Work out the finished part from the listing and answer in its coordinate system (mm). Round coordinates to 2 decimals unless told otherwise and drop trailing zeros. Loops run counter-clockwise (first coordinate to the right, second up) from the corner with the lowest first, then second, coordinate; pieces in that order, holes last. Notation, with made-up numbers: (-6.5, 71) - (43.5, 71) arc R15 cw to (43.5, 77) - close; hole circle Ø3 at (83, -25). An arc over 180 degrees is marked (long way). Use CSV: the item, a comma, the result in double quotes. Start each with the question number.
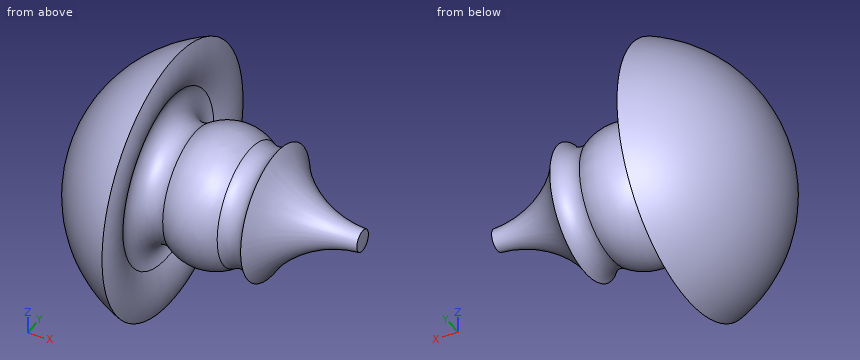
from build123d import *
from build123d.topology import SkipClean

# Parameters (mm, degrees)
SKETCH_3_R = 111.666392741


with BuildPart() as part:
    # 草圖1 → 旋轉1 (revolve)
    with BuildSketch(Plane.XY):
        with BuildLine():
            Line((0, 150), (0, -150))
            ThreePointArc((0, -150), (150, 0), (0, 150))
        make_face()
    revolve(axis=Axis((0, 150, 0), (0, -1, 0)))

    # 草圖2 → 除料-旋轉1 (revolve, cut)
    with SkipClean():  # the faces are left unmerged after this step: merging them gives an invalid solid
        with BuildSketch(Plane.XY, mode=Mode.PRIVATE) as cut_revolve_1_sk:
            with BuildLine():
                ThreePointArc((56.641005887, 148.905996075), (47.888974491, 120), (56.641005887, 91.094003925))
                ThreePointArc((56.641005887, 91.094003925), (54.142135624, 65.857864376), (28.905996075, 63.358994113))
                ThreePointArc((28.905996075, 63.358994113), (0, 72.111025509), (-28.905996075, 63.358994113))
                ThreePointArc((-28.905996075, 63.358994113), (-54.142135624, 65.857864376), (-56.641005887, 91.094003925))
                ThreePointArc((-56.641005887, 91.094003925), (-47.888974491, 120), (-56.641005887, 148.905996075))
                ThreePointArc((-56.641005887, 148.905996075), (-54.142135624, 174.142135624), (-28.905996075, 176.641005887))
                ThreePointArc((-28.905996075, 176.641005887), (0, 167.888974491), (28.905996075, 176.641005887))
                ThreePointArc((28.905996075, 176.641005887), (54.142135624, 174.142135624), (56.641005887, 148.905996075))
            make_face()
        revolve(cut_revolve_1_sk.sketch.rotate(Axis((0, 0, 0), (1, 0, 0)), 90), axis=Axis((0, 0, 0), (1, 0, 0)), mode=Mode.SUBTRACT)

    # 草圖3 → 除料-旋轉4 (revolve, cut)
    with SkipClean():  # the faces are left unmerged after this step: merging them gives an invalid solid
        with BuildSketch(Plane.XY, mode=Mode.PRIVATE) as cut_revolve_4_sk:
            with Locations((154.97116456, 123.10538907)):
                Circle(SKETCH_3_R)
        revolve(cut_revolve_4_sk.sketch.rotate(Axis((0, 0, 0), (1, 0, 0)), 90), axis=Axis((0, 0, 0), (1, 0, 0)), mode=Mode.SUBTRACT)


solid = part.part
Item 1: Find the intervals of material crossed by probe 1 along X at (y, z) = (4.5, 67.5); probe 2 along X at (y, z) = (1, 3); probe 3 along Y at (x, z) = (-16, 1), in increasing order. Write a range as [from, to].
Item 2: A cutting plane is placed at B-B (x = 48). Determine the outline of the cut face in (y, z).
Item 3: Each of these flat-tipped pins is pushed along its axis until it touches: pin 1 Ø4 at (x, z) = (-21.5, 29) entering from -Y; pin 2 Ø10 at (x, y) = (-13.5, -16.5) entering from -Z; pin 3 Ø8 at (x, z) = (-66.5, -39.5) entering from +Y. Where does it stop, or does it pass through?
Item 4: A cutting plane is placed at A-A (x = -40). Determine the outline of the cut face in (y, z), plus the area to 3 significant figures.
Result sheet:
1,probe 1,"[-133.88, -55.73], [-21.1, 21.1], [55.73, 58.05]"
1,probe 2,"[-149.97, 149.97]"
1,probe 3,"[-69.59, 69.59]"
2,outline,"circle Ø123.34 at (0, 0)"
3,pin 1,"y = -62.25"
3,pin 2,"z = -69.96"
3,pin 3,"y = 130.84"
4,outline,"circle Ø120 at (0, 0)"
4,area,"11,300 mm^2"
